Read the model definition and answer for the solid it produces. Units are mm, in the model's axes. A direction names the side the tool comes from. Coordinates: 2 decimals unless noted, no trailing zeros. Loops run counter-clockwise (first coordinate to the right, second up) from the corner with the lowest first, then second, coordinate; pieces in that order, holes last. Notation, with made-up numbers: (8, 76) -> (64, 76) arc R23 cw to (64, 94) -> close; hole circle Ø10 at (-2.75, 51.5). An arc over 180 degrees is marked (long way). Answer as a JSON object with one key per item and string values. Group by question number.
1) Section B-B, the plane x = 102.5 is taken. Give the vertices of the cut face in (y, z).
2) Section D-D, the plane x = 34 is taken. Give the vertices of the cut face in (y, z), plus the area to 3 significant figures.
3) Consider probe 1 along Y at (x, z) = (7, 0.9); probe 2 along X at (y, z) = (240, 0.4); probe 3 along Y at (x, z) = (61, 1.25). Determine where each line is inside the solid, lowest interval first. Write a range as [from, to].
4) Section A-A, the plane z = 6.25 is taken. Give the vertices of the cut face in (x, y).
5) Which of the six approach directions +Z, -Z, +X, -X, +Y, -Y give full straight-line access (tool end or side, diameter ignored) to faces 1 (the face through (55.5, 243, 6)), 2 (the face through (147.5, 241, 9)), 3 (the face through (99, 230.5, 9))?
6) Flat-ended cylindrical pins translate along their axes: P1, Ø5.5, axis at x = 7, y = 175, coming from the +Z side; P2, Ø2, axis at x = 90.5, y = 98, coming from the -Z side; P3, Ø1.5, axis at x = 92.5, z = 10, coming from the -Y side; P4, Ø6, axis at x = 77, z = 8, coming from the +Y side. Find the tip coordinate at first contact, or state that the pin passes through.
7) Section C-C, the plane y = 124 is taken. Give the vertices of the cut face in (x, z).
from build123d import *

# Parameters (mm, degrees)
SKETCH1_W           = 200
SKETCH1_H           = 250
BOSS_EXTRUDE1_DEPTH = 3
FILLET1_R           = 7
SKETCH2_W           = 89
SKETCH2_H           = 16.5
CUT_EXTRUDE2_DEPTH  = 3
EXTRUDE_THIN1_DEPTH = 8.25
SKETCH4_W           = 95
SKETCH4_H           = 19.5
BOSS_EXTRUDE2_DEPTH = 3
FILLET2_R           = 2
FILLET3_R           = 2
SKETCH5_R           = 1.65
CUT_EXTRUDE3_DEPTH  = 4
CHAMFER1_SIZE       = 1


with BuildPart() as part:
    # Sketch1 → Boss-Extrude1 (new body)
    with BuildSketch(Plane.XY):
        with Locations((100, 125)):
            Rectangle(SKETCH1_W, SKETCH1_H)
    extrude(amount=BOSS_EXTRUDE1_DEPTH)

    # Fillet1
    fillet1_edges = [part.edges().sort_by_distance(p)[0] for p in [
        (200, 0, 1.5),
        (0, 0, 1.5),
    ]]
    fillet(fillet1_edges, radius=FILLET1_R)

    # Sketch2 → Cut-Extrude2 (cut)
    with BuildSketch(Plane.XY):
        with Locations((100, 241.75)):
            Rectangle(SKETCH2_W, SKETCH2_H)
    extrude(amount=CUT_EXTRUDE2_DEPTH, mode=Mode.SUBTRACT)

    # Sketch3 → Extrude-Thin1 (add)
    with BuildSketch(Plane.XY.offset(3)):
        Polygon((144.5, 250), (144.5, 233.5), (55.5, 233.5), (55.5, 250), (52.5, 250), (52.5, 230.5), (147.5, 230.5), (147.5, 250), align=None)
    extrude(amount=EXTRUDE_THIN1_DEPTH)

    # Sketch4 → Boss-Extrude2 (add)
    with BuildSketch(Plane.XY.offset(11.25)):
        with Locations((100, 240.25)):
            Rectangle(SKETCH4_W, SKETCH4_H)
    extrude(amount=BOSS_EXTRUDE2_DEPTH)

    # Fillet2
    fillet2_edges = [part.edges().sort_by_distance(p)[0] for p in [
        (144.5, 233.5, 5.625),
        (55.5, 233.5, 5.625),
    ]]
    fillet(fillet2_edges, radius=FILLET2_R)

    # Fillet3
    fillet3_edges = [part.edges().sort_by_distance(p)[0] for p in [
        (52.5, 230.5, 8.625),
        (147.5, 230.5, 8.625),
    ]]
    fillet(fillet3_edges, radius=FILLET3_R)

    # Sketch5 → Cut-Extrude3 (cut, through all)
    with BuildSketch(Plane.XY.offset(3)):
        with Locations((12.5, 240)):
            Circle(SKETCH5_R)
        with Locations((187.5, 240)):
            Circle(SKETCH5_R)
        with Locations((7, 175)):
            Circle(SKETCH5_R)
        with Locations((7, 75)):
            Circle(SKETCH5_R)
        with Locations((61, 7)):
            Circle(SKETCH5_R)
        with Locations((139, 7)):
            Circle(SKETCH5_R)
        with Locations((193, 175)):
            Circle(SKETCH5_R)
        with Locations((193, 75)):
            Circle(SKETCH5_R)
    extrude(amount=-CUT_EXTRUDE3_DEPTH, mode=Mode.SUBTRACT)

    # Chamfer1
    chamfer1_edges = [part.edges().sort_by_distance(p)[0] for p in [
        (185.85, 240, 3),
        (5.35, 175, 3),
        (5.35, 75, 3),
        (59.35, 7, 3),
        (191.35, 75, 3),
        (191.35, 175, 3),
        (137.35, 7, 3),
        (10.85, 240, 3),
    ]]
    chamfer(chamfer1_edges, length=CHAMFER1_SIZE)


solid = part.part
Determined:
{
 "1": {"outline": "(0, 0) -> (233.5, 0) -> (233.5, 11.25) -> (250, 11.25) -> (250, 14.25) -> (230.5, 14.25) -> (230.5, 3) -> (0, 3) -> close"},
 "2": {"outline": "(0, 0) -> (250, 0) -> (250, 3) -> (0, 3) -> close", "area": "750 mm²"},
 "3": {"probe 1": "[0, 73.35], [76.65, 173.35], [176.65, 250]", "probe 2": "[0, 10.85], [14.15, 55.5], [144.5, 185.85], [189.15, 200]", "probe 3": "[0, 5.35], [8.65, 233.5]"},
 "4": {"outline": "(52.5, 232.5) arc R2 ccw to (54.5, 230.5) -> (145.5, 230.5) arc R2 ccw to (147.5, 232.5) -> (147.5, 250) -> (144.5, 250) -> (144.5, 235.5) arc R2 cw to (142.5, 233.5) -> (57.5, 233.5) arc R2 cw to (55.5, 235.5) -> (55.5, 250) -> (52.5, 250) -> close"},
 "5": {"face 1": "-Z, +Y", "face 2": "+Z, +X, +Y, -Y", "face 3": "+Z, +X, -X, -Y"},
 "6": {"P1": "z = 3", "P2": "z = 0", "P3": "y = 230.5", "P4": "y = 233.5"},
 "7": {"outline": "(0, 0) -> (200, 0) -> (200, 3) -> (0, 3) -> close"}
}
